```python
from build123d import *

# Parameters (mm, degrees)
EXTRUDE_3_DEPTH = 4


with BuildPart() as part:
    # ｽｹｯﾁ1 → ﾎﾞｽ - 押し出し3 (new body)
    with BuildSketch(Plane.XY):
        with BuildLine():
            Line((15, 6.5), (15, 2.5))
            Line((15, 2.5), (1.523471671, 2.5))
            Line((1.523471671, 2.5), (1.523471671, 1.982179121))
            ThreePointArc((1.523471671, 1.982179121), (2.242618913, 1.104835015), (2.5, 0))
            ThreePointArc((2.5, 0), (-1.104835015, -2.242618913), (-1.523471671, 1.982179121))
            Line((-1.523471671, 1.982179121), (-1.523471671, 2.5))
            Line((-1.523471671, 2.5), (-15, 2.5))
            Line((-15, 2.5), (-15, 6.5))
            Line((-15, 6.5), (-20, 6.5))
            Line((-20, 6.5), (-20, -28.5))
            Line((-20, -28.5), (-15, -33.5))
            Line((-15, -33.5), (-12, -33.5))
            Line((-12, -33.5), (-12, -31.5))
            Line((-12, -31.5), (-10, -31.5))
            Line((-10, -31.5), (-10, -33.5))
            Line((-10, -33.5), (0, -33.5))
            Line((0, -33.5), (10, -33.5))
            Line((10, -33.5), (10, -31.5))
            Line((10, -31.5), (12, -31.5))
            Line((12, -31.5), (12, -33.5))
            Line((12, -33.5), (15, -33.5))
            Line((15, -33.5), (20, -28.5))
            Line((20, -28.5), (20, 6.5))
            Line((20, 6.5), (15, 6.5))
        make_face()
        Polygon((-15, -27.27974657), (-15, -1.481890402), (-1.643206603, -15.516883287), align=None, mode=Mode.SUBTRACT)
        Polygon((-11.029061917, -26.739072938), (0, -17.026161792), (11.029061917, -26.739072938), align=None, mode=Mode.SUBTRACT)
        Polygon((15, -27.27974657), (1.643206603, -15.516883287), (15, -1.481890402), align=None, mode=Mode.SUBTRACT)
        Polygon((-8.526128996, -4.880410376), (8.526128996, -4.880410376), (0, -13.839458872), align=None, mode=Mode.SUBTRACT)
    extrude(amount=EXTRUDE_3_DEPTH)


solid = part.part
```
Read the model definition and answer for the solid it produces. Units are mm, in the model's axes. A direction names the side the tool comes from. Give positions to 0.01 mm unless a question says otherwise; leave off trailing zeros. Write each loop counter-clockwise with the first axis right and the second up, starting at its lowest first coordinate (ties: lowest second). Pieces come first, ordered by that corner, then holes. Notation, with made-up numbers: M 21,23.5 L 41,23.5 A17 ccw 41,46.5 Z; hole C -18.5,-22 d10. An arc over 180 degrees is marked long. Put each result on its own line as item: value. Start each with the question number.
1. The part is cut by section A-A, the plane x = 1. Give the vertices of the cut face in (y, z).
2. Each of these flat-tipped pins is pushed along its axis until it touches: pin 1 Ø0.6 at (y, z) = (-32.5, 2) entering from +X; pin 2 Ø2 at (y, z) = (-32.5, 3) entering from -X; pin 3 Ø1.6 at (y, z) = (-32.5, 2.5) entering from +X. Where does it stop, or does it pass through?
3. Consider line 1 along X through (y, z) = (4, 1.45); line 2 along X through (y, z) = (-9, 2.8); line 3 along X through (y, z) = (-3.5, 3.15). Determine where each line is inside the solid, lowest interval first.
4. The part is cut by section D-D, the plane x = -7.5. Give the vertices of the cut face in (y, z), and give its area (3 significant figures).
5. Which of the six approach directions +Z, -Z, +X, -X, +Y, -Y give full straight-line access (tool end or side, diameter ignored) to faces 4 (the flat face through (12, -32, 2)), 5 (the flat face through (-8, 2.5, 2)), 6 (the flat face through (4.32, -9.3, 1.97))?
6. The part is cut by section B-B, the plane x = 13. Give the vertices of the cut face in (y, z), and give its area (3 significant figures).
7. For a pull along X with two mould halves and no side action, classify faces 1 (the flat face through (0, -4, 0)), 2 (the flat face through (-17.5, -31, 2)), 3 (the flat face through (-8.415, -8.401, 1.972)) as released by +X, released by -X, zero draft, split by the parting line, or undercut.
8. The part is cut by section C-C, the plane y = -18.5. Give the vertices of the cut face in (x, z).
Final values:
1. outline: M -33.5,0 L -26.74,0 L -26.74,4 L -33.5,4 Z; M -17.91,0 L -12.79,0 L -12.79,4 L -17.91,4 Z; M -4.88,0 L -2.29,0 L -2.29,4 L -4.88,4 Z
2. pin 1: stops at x = 16.3
2. pin 2: stops at x = -17
2. pin 3: stops at x = 16.8
3. line 1: x = -20 to -15, 15 to 20
3. line 2: x = -20 to -15, -7.85 to -4.61, 4.61 to 7.85, 15 to 20
3. line 3: x = -20 to -15, -13.08 to 13.08, 15 to 20
4. outline: M -33.5,0 L -26.74,0 L -26.74,4 L -33.5,4 Z; M -23.63,0 L -20.67,0 L -20.67,4 L -23.63,4 Z; M -9.36,0 L -5.96,0 L -5.96,4 L -9.36,4 Z; M -4.88,0 L 2.5,0 L 2.5,4 L -4.88,4 Z
4. area: 82.0 mm²
5. face 4: +Z, -Z, -Y
5. face 5: +Z, -Z, +Y
5. face 6: +Z, -Z
6. outline: M -33.5,0 L -25.52,0 L -25.52,4 L -33.5,4 Z; M -3.58,0 L 2.5,0 L 2.5,4 L -3.58,4 Z
6. area: 56.3 mm²
7. face 1: zero draft
7. face 2: released by -X
7. face 3: undercut
8. outline: M -20,0 L -15,0 L -15,4 L -20,4 Z; M -5.03,0 L -1.67,0 L -1.67,4 L -5.03,4 Z; M 1.67,0 L 5.03,0 L 5.03,4 L 1.67,4 Z; M 15,0 L 20,0 L 20,4 L 15,4 Z
